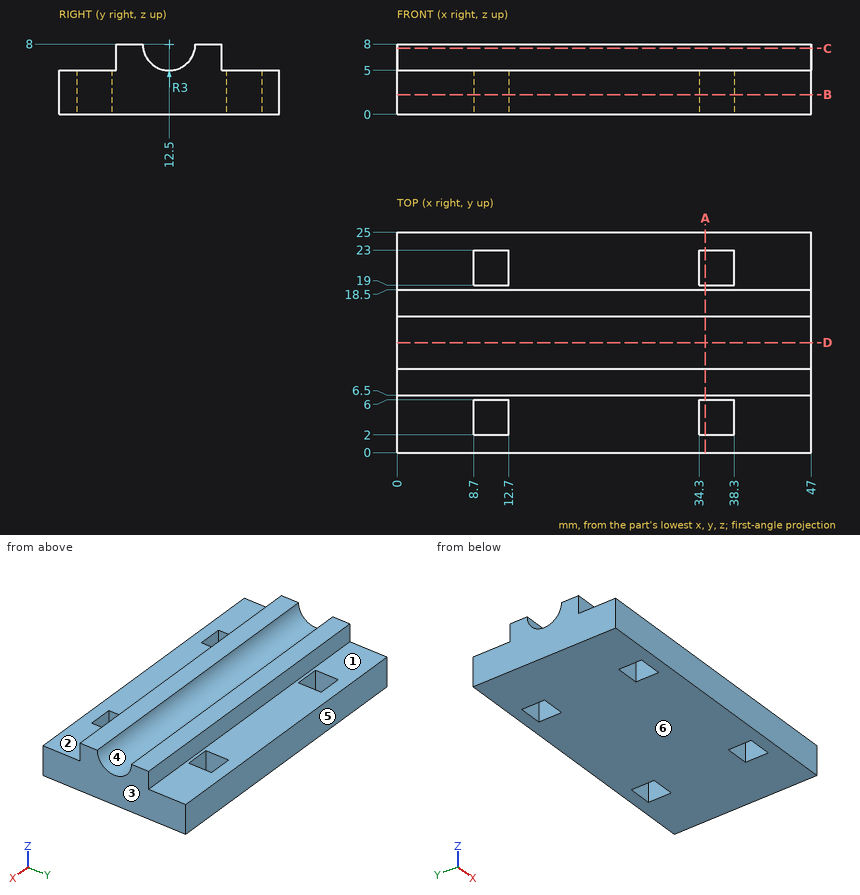
Could you check a few things on this drawing? It's one solid part, dimensions in mm from its lowest x, y, z. A direction names the side the tool comes from. Coordinates: 2 decimals unless noted, no trailing zeros. Write each loop counter-clockwise with the first axis right and the second up, starting at its lowest first coordinate (ties: lowest second). Pieces come first, ordered by that corner, then holes. Notation, with made-up numbers: (39, 46.25) - (89, 46.25) arc R20 ccw to (89, 78.25) - close; hole circle Ø4 at (56, 53). An arc over 180 degrees is marked (long way). Put each result on its own line as item: value. Start each with the question number.
Q1. Which directions (+Z, -Z, +X, -X, +Y, -Y) give clear straight access to the entire face, cutting with the end or side of a thin tool? Please do the marked faces 1, 2 and 3.
Q2. Please list where these lines run through material, in increasing order: L1, parallel to Y at x = 38, z = 4.75; L2, parallel to Z at x = 14.5, y = 1.75; L3, parallel to Y at x = 42, z = 6.75.
Q3. I want a section at C-C on z = 7.5. Write out the boundary of the cut face in (x, y).
Q4. I want a section at D-D on y = 12.5. Write out the boundary of the cut face in (x, z), plus the area to 3 significant figures.
Q5. I want a section at A-A on x = 35. Write out the boundary of the cut face in (y, z), plus the area to 3 significant figures.
Q6. Thinking about a two-plate mould opening in Y: for the marked faces 4, 5 and 6, which applies, pulls with the +Y half, pulls with the -Y half, needs draft (parallel to the pull), parting line crosses it, or undercut?
Q7. I want a section at B-B on z = 2.25. Write out the boundary of the cut face in (x, y).
Q8. I'm going to push a flat-ended pin straight in: P1, Ø2.5, axis at x = 34, z = 7, coming from the -Y side. Where does the tip first touch, or does it pass through?
Checks:
1. face 1: +Z, +X, -X, +Y
1. face 2: +Z, +X, -X, -Y
1. face 3: +Z, -Z, +X, +Y, -Y
2. L1: 0 to 2, 6 to 19, 23 to 25
2. L2: 0 to 5
2. L3: 6.5 to 9.77, 15.23 to 18.5
3. outline: (0, 6.5) - (47, 6.5) - (47, 9.54) - (0, 9.54) - close; (0, 15.46) - (47, 15.46) - (47, 18.5) - (0, 18.5) - close
4. outline: (0, 0) - (47, 0) - (47, 5) - (0, 5) - close
4. area: 235 mm²
5. outline: (0, 0) - (2, 0) - (2, 5) - (0, 5) - close; (6, 0) - (19, 0) - (19, 5) - (18.5, 5) - (18.5, 8) - (15.5, 8) arc R3 cw to (9.5, 8) - (6.5, 8) - (6.5, 5) - (6, 5) - close; (23, 0) - (25, 0) - (25, 5) - (23, 5) - close
5. area: 107 mm²
6. face 4: undercut
6. face 5: pulls with the +Y half
6. face 6: needs draft
7. outline: (0, 0) - (47, 0) - (47, 25) - (0, 25) - close; hole (8.7, 2) - (12.7, 2) - (12.7, 6) - (8.7, 6) - close; hole (8.7, 19) - (12.7, 19) - (12.7, 23) - (8.7, 23) - close; hole (34.3, 2) - (38.3, 2) - (38.3, 6) - (34.3, 6) - close; hole (34.3, 19) - (38.3, 19) - (38.3, 23) - (34.3, 23) - close
8. P1: y = 6.5
